from build123d import *

# Parameters (mm, degrees)
SKETCH1_W                 = 72
SKETCH1_H                 = 45
BOSS_EXTRUDE1_DEPTH       = 9
SKETCH3_W                 = 27
SKETCH3_H                 = 7
BOSS_EXTRUDE3_DEPTH       = 9
SKETCH4_W                 = 27
SKETCH4_H                 = 7
BOSS_EXTRUDE4_DEPTH       = 9
SKETCH5_W                 = 3
SKETCH5_H                 = 18
CUT_EXTRUDE1_DEPTH        = 9
BOSS_EXTRUDE5_DEPTH       = 9
FILLET1_R                 = 4.5
F_4_0MM_DOWEL_HOLE1_D     = 4
F_3_0MM_DOWEL_HOLE1_D     = 3
SKETCH12_W                = 21
SKETCH12_H                = 6
CUT_EXTRUDE3_DEPTH        = 9
CHAMFER1_SIZE             = 3
F_3_0MM_DOWEL_HOLE2_D     = 3
F_3_0MM_DOWEL_HOLE2_DEPTH = 18
F_3_0MM_DOWEL_HOLE2_TIP   = 0.901290929
SKETCH16_W                = 27
SKETCH16_H                = 33
SKETCH16_W_2              = 18
SKETCH16_H_2              = 18
CUT_EXTRUDE4_DEPTH        = 9
BOSS_EXTRUDE7_DEPTH       = 9
BOSS_EXTRUDE8_DEPTH       = 9
BOSS_EXTRUDE10_DEPTH      = 9


with BuildPart() as part:
    # Sketch1 → Boss-Extrude1 (new body)
    with BuildSketch(Plane(origin=(0, 0, 0), x_dir=(1, 0, 0), z_dir=(0, 1, 0))):
        with Locations((36, 22.5)):
            Rectangle(SKETCH1_W, SKETCH1_H)
    extrude(amount=BOSS_EXTRUDE1_DEPTH)

    # Sketch3 → Boss-Extrude3 (add)
    with BuildSketch(Plane(origin=(0, 0, 0), x_dir=(1, 0, 0), z_dir=(0, 1, 0))):
        with Locations((82.5, 28.5)):
            Rectangle(SKETCH3_W, SKETCH3_H)
    extrude(amount=BOSS_EXTRUDE3_DEPTH)

    # Sketch4 → Boss-Extrude4 (add)
    with BuildSketch(Plane(origin=(0, 0, 0), x_dir=(1, 0, 0), z_dir=(0, 1, 0))):
        with Locations((82.5, 3.5)):
            Rectangle(SKETCH4_W, SKETCH4_H)
    extrude(amount=BOSS_EXTRUDE4_DEPTH)

    # Sketch5 → Cut-Extrude1 (cut)
    with BuildSketch(Plane(origin=(0, 9, 0), x_dir=(1, 0, 0), z_dir=(0, 1, 0))):
        with Locations((70.5, 16)):
            Rectangle(SKETCH5_W, SKETCH5_H)
    extrude(amount=-CUT_EXTRUDE1_DEPTH, mode=Mode.SUBTRACT)

    # Sketch6 → Boss-Extrude5 (add)
    with BuildSketch(Plane(origin=(0, 9, 0), x_dir=(1, 0, 0), z_dir=(0, 1, 0))):
        Polygon((72, 45), (72, 32), (85, 32), align=None)
    extrude(amount=-BOSS_EXTRUDE5_DEPTH)

    # Fillet1
    fillet1_edges = [part.edges().sort_by_distance(p)[0] for p in [
        (0, 0, -22.5),
        (0, 9, -22.5),
        (72, 4.5, -45),
        (85, 4.5, -32),
        (96, 0, -3.5),
        (96, 9, -3.5),
        (96, 0, -28.5),
        (96, 9, -28.5),
    ]]
    fillet(fillet1_edges, radius=FILLET1_R - 0.0001)  # a hair under: the kernel refuses the full size

    # Ø4.0mm Dowel Hole1 (through all)
    with Locations(Plane(origin=(0, 0, -45), x_dir=(-1, 0, 0), z_dir=(0, 0, -1))):
        with Locations((-4.5, 4.5)):
            Hole(F_4_0MM_DOWEL_HOLE1_D / 2)

    # Ø3.0mm Dowel Hole1 (through all)
    with Locations(Plane.XY):
        with Locations((91.5, 4.5)):
            Hole(F_3_0MM_DOWEL_HOLE1_D / 2)

    # Sketch12 → Cut-Extrude3 (cut)
    with BuildSketch(Plane(origin=(0, 9, 0), x_dir=(1, 0, 0), z_dir=(0, 1, 0))):
        with Locations((58.5, 36)):
            Rectangle(SKETCH12_W, SKETCH12_H)
    extrude(amount=-CUT_EXTRUDE3_DEPTH, mode=Mode.SUBTRACT)

    # Chamfer1
    chamfer1_edges = [part.edges().sort_by_distance(p)[0] for p in [
        (48, 0, -36),
        (58.5, 0, -39),
        (69, 0, -36),
        (58.5, 0, -33),
        (48, 9, -36),
        (58.5, 9, -33),
        (69, 9, -36),
        (58.5, 9, -39),
    ]]
    chamfer(chamfer1_edges, length=CHAMFER1_SIZE)

    # Ø3.0mm Dowel Hole2
    with Locations(Plane(origin=(0, 0, -45), x_dir=(-1, 0, 0), z_dir=(0, 0, -1))):
        with Locations((-58, 4.5)):
            Hole(F_3_0MM_DOWEL_HOLE2_D / 2, depth=F_3_0MM_DOWEL_HOLE2_DEPTH)
            with Locations((0, 0, -(F_3_0MM_DOWEL_HOLE2_DEPTH + F_3_0MM_DOWEL_HOLE2_TIP / 2))):  # 118° drill point
                Cone(0, F_3_0MM_DOWEL_HOLE2_D / 2, F_3_0MM_DOWEL_HOLE2_TIP, mode=Mode.SUBTRACT)

    # Sketch16 → Cut-Extrude4 (cut)
    with BuildSketch(Plane(origin=(0, 9, 0), x_dir=(1, 0, 0), z_dir=(0, 1, 0))):
        with Locations((25.5, 22.5)):
            Rectangle(SKETCH16_W, SKETCH16_H)
        with Locations((54, 15)):
            Rectangle(SKETCH16_W_2, SKETCH16_H_2)
    extrude(amount=-CUT_EXTRUDE4_DEPTH, mode=Mode.SUBTRACT)

    # Sketch17 → Boss-Extrude7 (add)
    with BuildSketch(Plane(origin=(0, 9, 0), x_dir=(1, 0, 0), z_dir=(0, 1, 0))):
        Polygon((39, 6), (41.321871898, 7.899713371), (14.321871898, 40.899713371), (12, 39), (9.678128102, 37.100286629), (36.678128102, 4.100286629), align=None)
    extrude(amount=-BOSS_EXTRUDE7_DEPTH)

    # Sketch18 → Boss-Extrude8 (add)
    with BuildSketch(Plane(origin=(0, 9, 0), x_dir=(1, 0, 0), z_dir=(0, 1, 0))):
        Polygon((12, 6), (14.321871898, 4.100286629), (41.321871898, 37.100286629), (39, 39), (36.678128102, 40.899713371), (9.678128102, 7.899713371), align=None)
    extrude(amount=-BOSS_EXTRUDE8_DEPTH)

    # Sketch19 → Boss-Extrude10 (add)
    with BuildSketch(Plane(origin=(0, 9, 0), x_dir=(1, 0, 0), z_dir=(0, 1, 0))):
        Polygon((58.242640687, 15), (54, 10.757359313), (58.757359313, 6), (63, 6), (63, 10.242640687), align=None)
        Polygon((45, 19.757359313), (49.757359313, 15), (54, 19.242640687), (49.242640687, 24), (45, 24), align=None)
        Polygon((54, 19.242640687), (58.242640687, 15), (63, 19.757359313), (63, 24), (58.757359313, 24), align=None)
        Polygon((45, 10.242640687), (45, 6), (49.242640687, 6), (54, 10.757359313), (49.757359313, 15), align=None)
        Polygon((49.757359313, 15), (54, 10.757359313), (58.242640687, 15), (54, 19.242640687), align=None)
    extrude(amount=-BOSS_EXTRUDE10_DEPTH)


solid = part.part
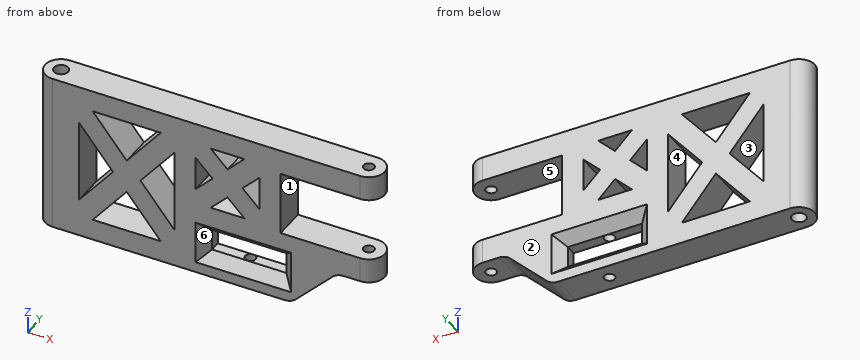
For this review, take the finished solid that the model builds, in its own axes (mm). Face numbers are marked on the shaded views. A direction names the side the tool comes from. Give positions to 0.01 mm unless a question says otherwise; leave off trailing zeros. Loops run counter-clockwise (first coordinate to the right, second up) from the corner with the lowest first, then second, coordinate; pieces in that order, holes last.
Item 1: Take a section at C-C, the plane x = 37. State the section outline as (y, z) points.
Item 2: Draft analysis for pull direction X (two halves, no side actions). For the marked faces 1, 2 and 3, state which applies: +X half, -X half, draft (parallel to the pull), parting line (faces both ways), or undercut.
Item 3: Tool access review of the marked faces 4, 5 and 6: name each direction out of +Z, -Z, +X, -X, +Y, -Y from which nothing blocks a thin tool from reaching the whole face with its end or side.
Item 4: For line 1 along X through (y, z) = (5.5, -40.5); line 2 along X through (y, z) = (2.75, -35); line 3 along Z through (x, y) = (48.5, 2.25), list the stretches that pass through material, from the lowest coordinate up.
Item 5: Take a section at B-B, the plane z = -41. Give the number of separate pieces and of enclosed holes in the cut face, and give its area (3 significant figures).
Item 6: Insertion check: pin 1 (4.5 mm diameter, centred on y = 5, z = -19.5, fed in from +X); pin 2 (3.5 mm diameter, centred on x = 91.5, y = 4.5, fed in from -Z); pin 3 (4 mm diameter, centred on y = 1.5, z = -16, fed in from -X); pin 4 (2.5 mm diameter, centred on x = 91.5, y = 4.5, fed in from -Z). Each pin has a flat end and moves straight along its axis. Give the tip position at first contact, or say it passes through.
Item 7: Take a section at A-A, the plane x = 78.5. State the section outline as (y, z) points, and give its area (4 significant figures).
Calculated:
1. outline: (0, -45) - (9, -45) - (9, -31.82) - (0, -31.82) - close; (0, -13.18) - (9, -13.18) - (9, 0) - (0, 0) - close
2. face 1: +X half
2. face 2: draft
2. face 3: undercut
3. face 4: +Y, -Y
3. face 5: +X, +Y, -Y
3. face 6: -Y
4. line 1: x = 0.11 to 2.77, 6.23 to 56.88, 59.12 to 76.5
4. line 2: x = 0.35 to 3.53, 5.47 to 19.15, 31.85 to 47.75, 69.25 to 82
4. line 3: z = -45 to -39.75, -32.25 to -16.26, -13.74 to 0
5. separate pieces: 1
5. enclosed holes: 2
5. area: 604 mm2
6. pin 1: stops at x = 69
6. pin 2: stops at z = -32
6. pin 3: stops at x = 0.11
6. pin 4: passes through
7. outline: (0, -38.5) - (9, -38.5) - (9, -25) - (0, -25) - close; (0, -7) - (9, -7) - (9, 0) - (0, 0) - close
7. area: 184.5 mm2
